Could you check a few things on this model? Use its own coordinates, in mm. A direction names the side the tool comes from. Give positions to 0.01 mm unless a question says otherwise; leave off trailing zeros. Order: outer loops, then holes, each group sorted by start corner. A loop starts at its lowest first (then second) coordinate and runs counter-clockwise, first axis right, second up. Notation, with made-up numbers: (-13.75, 47) -> (4.25, 47) arc R20 cw to (4.25, 52) -> close; hole circle Ø6 at (40.5, 67). An arc over 180 degrees is marked (long way). Write each question's results on one line, items separated by ' | '.
Autodesk Inventor part; units mm, degrees
ref_plane "Work Plane1" through (91.5, 0, 0) normal (-1, 0, 0) x (0, 0, 1)
ref_plane "YZ Plane" through (0, 0, 0) normal (1, 0, 0) x (0, 1, 0)
ref_plane "XZ Plane" through (0, 0, 0) normal (0, 1, 0) x (-1, 0, 0)
sketch "Sketch1" plane through (0, 0, 0) normal (0, 0, 1) x (1, 0, 0)
  line L0 (0, 0) -> (183, 0)
  line L1 (183, 0) -> (183, 115)
  line L2 (183, 115) -> (0, 115)
  line L3 (0, 115) -> (0, 0)
  dimension "d0" = 183
  dimension "d1" = 115
extrude "Extrusion1" add sketch "Sketch1" along normal blind 12
sketch "Sketch2" plane through (0, 115, 0) normal (0, 1, 0) x (1, 0, 0)
  line L0 (0, 0) -> (0, -12)
  line L1 (0, -12) -> (183, -12)
  line L2 (183, 0) -> (0, 0)
  line L3 (7.4669, -2.4521) -> (177.6982, -2.4521)
  line L4 (177.8669, -9.25) -> (7.4669, -9.25)
  line L5 (7.4669, -6.2521) -> (7.4669, -2.4521)
  line L6 (7.4669, -9.2521) -> (7.4669, -9.25)
  line L7 (177.6982, -6.25) -> (177.6982, -2.4521)
  line L8 (7.4669, -9.2521) -> (4.4669, -9.2521)
  line L9 (4.4669, -9.2521) -> (4.4669, -6.2521)
  line L10 (4.4669, -6.2521) -> (7.4669, -6.2521)
  line L11 (177.8669, -9.25) -> (180.8669, -9.25)
  line L12 (180.8669, -9.25) -> (180.8669, -6.25)
  line L13 (180.8669, -6.25) -> (177.6982, -6.25)
  point P0 (0, -6)
  point P1 (0, -6)
  point P2 (0, -6)
  point P3 (0, -6)
  point P4 (91.5, -2.4521)
  point P5 (91.5, 0)
  point P6 (0, -6)
  point P7 (7.3, -9.25)
  dimension "d75" = 170.4
  dimension "d76" = 6.8
  dimension "d122" = 2.75
  dimension "d123" = 6.8
  dimension "d131" = 3
  dimension "d132" = 3
  dimension "d134" = 3
  dimension "d135" = 3
  dimension "d136" = 90
ref_plane "Work Plane1" through (91.5, 0, 0) normal (-1, 0, 0) x (0, 0, 1)
sketch "Sketch6" plane through (91.5, 0, 0) normal (-1, 0, 0) x (0, 0, 1)
  point P0 (0, 115)
  point P1 (0, 101)
sketch "Sketch7" plane through (0, 0, 0) normal (0, 0, -1) x (-1, 0, 0)
  line L0 (-146.5, 112) -> (-36.5, 112)
  line L1 (-36.5, 112) -> (-36.5, 115)
  line L2 (-36.5, 115) -> (-146.5, 115)
  line L3 (-146.5, 115) -> (-146.5, 112)
  line L4 (-183, 115) -> (0, 115)
  point P0 (0, 0)
  point P1 (-91.5, 115)
  point P2 (-91.5, 115)
  dimension "d34" = 110
  dimension "d35" = 3
sketch "Sketch14" plane through (0, 0, 12) normal (-1, 0, 0) x (0, 0, 1)
  line L0 (-9, 101) -> (-11, 101)
  line L1 (-11, 101) -> (-12, 98.8551)
  line L2 (-12, 0) -> (-12, 115)
  line L3 (-9, 101) -> (-6.8161, 101)
  line L4 (-9, 101) -> (-11, 101)
  line L5 (-9, 101) -> (-9, 98.8551)
sketch "Sketch15" plane through (183, 0, 12) normal (1, 0, 0) x (0, 0, -1)
  line L0 (11, 101) -> (12, 98.8551)
  line L1 (9, 101) -> (11, 101)
  line L2 (12, 115) -> (12, 0)
  point P0 (12, 0)
extrude "Extrusion15" cut sketch "Sketch2" against normal blind 110
sketch "Sketch18" plane through (0, 0, 12) normal (0, 0, 1) x (1, 0, 0)
  line L0 (14.75, 98.5) -> (168.25, 98.5)
  line L1 (168.25, 98.5) -> (168.25, 14.5)
  line L2 (168.25, 14.5) -> (14.75, 14.5)
  line L3 (14.75, 14.5) -> (14.75, 98.5)
  line L4 (183, 0) -> (0, 0)
  line L5 (0, 115) -> (183, 115)
  point P0 (91.5, 98.5)
  point P1 (91.5, 115)
  dimension "d88" = 153.5
  dimension "d89" = 84
  dimension "d90" = 14.5
sketch "Sketch19" plane through (0, 115, 0) normal (0, 1, 0) x (1, 0, 0)
  line L0 (183, 0) -> (0, 0)
  line L1 (7.4669, -2.4521) -> (177.6982, -2.4521)
  line L2 (129.8823, -2.4521) -> (129.8823, 0)
  line L3 (53.4515, -2.4521) -> (53.4515, 0)
  line L4 (129.8823, -2.4521) -> (53.4515, -2.4521)
  line L5 (53.4515, 0) -> (129.8823, 0)
  point P0 (53.4515, 0)
  point P1 (53.4515, -2.4521)
extrude "Extrusion16" cut sketch "Sketch19" against normal blind 5
sketch "Sketch21" plane through (0, 0, 0) normal (0, 0, -1) x (-1, 0, 0)
  line L0 (-129.8823, 110) -> (-53.4515, 110)
  line L1 (0, 115) -> (-183, 115)
  line L2 (-53.4515, 110) -> (0, 110)
  line L3 (0, 110) -> (0, 115)
  line L4 (0, 115) -> (-53.4515, 115)
  line L5 (-53.4515, 115) -> (-53.4515, 110)
  line L6 (-183, 0) -> (-183, 115)
  line L7 (-183, 115) -> (-129.8898, 115)
  line L8 (-129.8898, 115) -> (-129.8898, 110)
  line L9 (-129.8898, 110) -> (-183, 110)
  line L10 (-183, 110) -> (-183, 115)
  point P0 (0, 0)
  point P1 (-129.8898, 115)
extrude "Extrusion17" add sketch "Sketch21" along normal blind 2.25
sketch "Sketch22" plane through (0, 0, 12) normal (-1, 0, 0) x (0, 0, 1)
  line L0 (-14.25, 115) -> (0, 115)
  line L1 (-14.25, 115) -> (-9.25, 115)
  line L2 (-9.25, 115) -> (-9.25, 110)
  line L3 (-12, 110) -> (-14.25, 110)
  line L4 (-9.25, 110) -> (-14.25, 110)
  circle A0 centre (-11.75, 112.5) radius 1.6
  point P0 (-12, 0)
  dimension "d95" = 5
  dimension "d96" = 5
  dimension "d97" = 90
  dimension "d98" = 3.2
extrude "Extrusion18" cut sketch "Sketch22" against normal through all
sketch "Sketch23" plane through (0, 0, 0) normal (0, 0, -1) x (-1, 0, 0)
  line L0 (-36.5, 115) -> (-146.5, 115)
  line L1 (-183, 110) -> (-129.8898, 110)
  line L2 (-133, 110) -> (-68, 110)
  line L3 (-68, 110) -> (-68, 60.5)
  line L4 (-68, 60.5) -> (-133, 60.5)
  line L5 (-133, 60.5) -> (-133, 110)
  line L6 (0, 110) -> (0, 0)
  line L7 (-183, 0) -> (-183, 110)
  dimension "d101" = 49.5
  dimension "d102" = 68
  dimension "d103" = 50
extrude "Extrusion19" cut sketch "Sketch23" against normal up to surface (9.25 mm away)
sketch "Sketch24" plane through (0, 0, 0) normal (0, 0, -1) x (-1, 0, 0)
  line L0 (-57.7492, 99.1931) -> (-47.7492, 99.1931)
  line L1 (-47.7492, 99.1931) -> (-47.7492, 89.1931)
  line L2 (-47.7492, 89.1931) -> (-57.7492, 89.1931)
  line L3 (-57.7492, 89.1931) -> (-57.7492, 99.1931)
  line L4 (-11.7492, 99.1931) -> (-1.7492, 99.1931)
  line L5 (-1.7492, 99.1931) -> (-1.7492, 89.1931)
  line L6 (-1.7492, 89.1931) -> (-11.7492, 89.1931)
  line L7 (-11.7492, 89.1931) -> (-11.7492, 99.1931)
  line L8 (-57.7492, 21.1931) -> (-47.7492, 21.1931)
  line L9 (-47.7492, 21.1931) -> (-47.7492, 11.1931)
  line L10 (-47.7492, 11.1931) -> (-57.7492, 11.1931)
  line L11 (-57.7492, 11.1931) -> (-57.7492, 21.1931)
  line L12 (-11.7492, 21.1931) -> (-1.7492, 21.1931)
  line L13 (-1.7492, 21.1931) -> (-1.7492, 11.1931)
  line L14 (-1.7492, 11.1931) -> (-11.7492, 11.1931)
  line L15 (-11.7492, 11.1931) -> (-11.7492, 21.1931)
  point P0 (0, 0)
  point P1 (-57.7492, 16.1931)
  point P2 (-57.7492, 94.1931)
  point P3 (-6.7492, 11.1931)
  point P4 (-6.7492, 99.1931)
  dimension "d108" = 10
  dimension "d109" = 10
  dimension "d110" = 10
  dimension "d111" = 10
  dimension "d112" = 10
  dimension "d113" = 10
  dimension "d114" = 10
  dimension "d115" = 10
  dimension "d116" = 56
  dimension "d118" = 88
  dimension "d137" = 88
extrude "Extrusion20" add sketch "Sketch24" along normal blind 5
extrude "Extrusion21" cut sketch "Sketch18" against normal blind 10
chamfer "Chamfer1" distance 1 angle 45 2 edges at (26.7257, 110, -2.25) (156.4449, 110, -2.25)
properties part number "stojan - správná verze"
Q1. For faces 4 (the flat face through (7.467, 61, 4)), 5 (the flat face through (11.749, 94, -2)), 6 (the flat face through (1.749, 94, -2)), which set-ups out of +Z, -Z, +X, -X, +Y, -Y let a thin tool reach every point of the face, with its end or its side?
Here are the results:
face 4: +Y | face 5: -Z, -Y | face 6: -Z, -X, -Y
Q2. I'm going to push flat-ended pins straight in: pin 1 Ø0.9 at (y, z) = (68, 7.5) entering from -X; pin 2 Ø1 at (x, y) = (156.5, 44) entering from -Z; pin 3 Ø1.5 at (x, y) = (70.5, 84.5) entering from -Z; pin 4 Ø2.5 at (x, z) = (54, -3) entering from -Y. Where does each tip first touch, or does it pass through?
Here are the results:
pin 1: stops at x = 0 | pin 2: stops at z = 0 | pin 3: passes through | pin 4: stops at y = 11.19
Q3. Suppose I cut it at B-B on x = 81. Please give me the cut outline in (y, z), and give its area (3 significant figures).
Here are the results:
outline: (0, 0) -> (60.5, 0) -> (60.5, 2) -> (14.5, 2) -> (14.5, 2.45) -> (5, 2.45) -> (5, 9.25) -> (14.5, 9.25) -> (14.5, 12) -> (0, 12) -> close; (98.5, 9.25) -> (115, 9.25) -> (115, 12) -> (98.5, 12) -> close | area: 247 mm²
Q4. Suppose I cut it at A-A on x = 153. Please give me the cut outline in (y, z).
Here are the results:
outline: (0, 0) -> (110, 0) -> (110, -1.25) -> (111, -2.25) -> (115, -2.25) -> (115, 2.45) -> (98.5, 2.45) -> (98.5, 2) -> (14.5, 2) -> (14.5, 2.45) -> (5, 2.45) -> (5, 9.25) -> (14.5, 9.25) -> (14.5, 12) -> (0, 12) -> close; (98.5, 9.25) -> (115, 9.25) -> (115, 12) -> (98.5, 12) -> close; hole circle Ø3.2 at (112.5, 0.25)
Q5. Thinking about a two-plate mould opening in Z: for faces 1 (the flat face through (7, 94, -5)), 2 (the flat face through (150.2, 110, -0.2)), 3 (the flat face through (177.698, 61, 4)), which applies, +Z half, -Z half, draft (parallel to the pull), parting line (faces both ways), or undercut?
Here are the results:
face 1: -Z half | face 2: draft | face 3: undercut
Q6. I need wall thicknesses on line 1 along Z through (x, y) = (18.5, 112.5); line 2 along Y through (x, z) = (56.5, -1.5); line 3 along X through (y, z) = (94, 10.25). Which ranges of each line are inside material? Lowest first, please.
Here are the results:
line 1: z = -2.25 to -1.35, 1.85 to 2.45, 9.25 to 12 | line 2: y = 11.19 to 21.19, 89.19 to 99.19 | line 3: x = 0 to 14.75, 168.25 to 183
